from build123d import *

# Parameters (mm, degrees)
RESSALTO_EXTRUS_O2_DEPTH = 3
RESSALTO_EXTRUS_O3_DEPTH = 3
ESBO_O4_R                = 1.65
CORTE_EXTRUS_O2_DEPTH    = 55.465328173


with BuildPart() as part:
    # Esboço1 → Ressalto-extrusão2 (new body)
    with BuildSketch(Plane.XY):
        Polygon((-23.89, 48.854271798), (-23.89, 4.854271798), (-18.042684332, 4.854271798), (3.957315668, 4.854271798), (18.042684332, 4.854271798), (23.89, 4.854271798), (23.89, 48.854271798), align=None)
        Polygon((19.113248654, 42), (16.226497308, 47), (22, 47), (22, 42), align=None, mode=Mode.SUBTRACT)
        Polygon((-16.226497308, 8), (-22, 8), (-22, 13), (-19.113248654, 13), align=None, mode=Mode.SUBTRACT)
        Polygon((-8.113248654, 19.947441117), (-5.226497308, 14.947441117), (-8.113248654, 9.947441117), (-13.886751346, 9.947441117), (-16.773502692, 14.947441117), (-13.886751346, 19.947441117), align=None, mode=Mode.SUBTRACT)
        Polygon((-19.113248654, 16), (-22, 16), (-22, 26), (-19.113248654, 26), (-16.226497308, 21), align=None, mode=Mode.SUBTRACT)
        Polygon((-2.886751346, 13), (2.886751346, 13), (5.773502692, 8), (-5.773502692, 8), align=None, mode=Mode.SUBTRACT)
        Polygon((22, 8), (16.226497308, 8), (19.113248654, 13), (22, 13), align=None, mode=Mode.SUBTRACT)
        Polygon((13.886751346, 19.947441117), (16.773502692, 14.947441117), (13.886751346, 9.947441117), (8.113248654, 9.947441117), (5.226497308, 14.947441117), (8.113248654, 19.947441117), align=None, mode=Mode.SUBTRACT)
        Polygon((-2.886751346, 26), (2.886751346, 26), (5.773502692, 21), (2.886751346, 16), (-2.886751346, 16), (-5.773502692, 21), align=None, mode=Mode.SUBTRACT)
        Polygon((22, 16), (19.113248654, 16), (16.226497308, 21), (19.113248654, 26), (22, 26), align=None, mode=Mode.SUBTRACT)
        Polygon((-19.113248654, 29), (-22, 29), (-22, 39), (-19.113248654, 39), (-16.226497308, 34), align=None, mode=Mode.SUBTRACT)
        Polygon((-8.113248654, 33.044060566), (-5.226497308, 28.044060566), (-8.113248654, 23.044060566), (-13.886751346, 23.044060566), (-16.773502692, 28.044060566), (-13.886751346, 33.044060566), align=None, mode=Mode.SUBTRACT)
        Polygon((-19.113248654, 42), (-22, 42), (-22, 47), (-16.226497308, 47), align=None, mode=Mode.SUBTRACT)
        Polygon((-8.113248654, 46.140680015), (-5.226497308, 41.140680015), (-8.113248654, 36.140680015), (-13.886751346, 36.140680015), (-16.773502692, 41.140680015), (-13.886751346, 46.140680015), align=None, mode=Mode.SUBTRACT)
        Polygon((-2.886751346, 39), (2.886751346, 39), (5.773502692, 34), (2.886751346, 29), (-2.886751346, 29), (-5.773502692, 34), align=None, mode=Mode.SUBTRACT)
        Polygon((13.886751346, 32.995750841), (16.773502692, 27.995750841), (13.886751346, 22.995750841), (8.113248654, 22.995750841), (5.226497308, 27.995750841), (8.113248654, 32.995750841), align=None, mode=Mode.SUBTRACT)
        Polygon((19.113248654, 39), (22, 39), (22, 29), (19.113248654, 29), (16.226497308, 34), align=None, mode=Mode.SUBTRACT)
        Polygon((-5.801394324, 47.096619449), (5.801394324, 47.096619449), (2.858859713, 42), (-2.858859713, 42), align=None, mode=Mode.SUBTRACT)
        Polygon((13.886751346, 46.044060566), (16.773502692, 41.044060566), (13.886751346, 36.044060566), (8.113248654, 36.044060566), (5.226497308, 41.044060566), (8.113248654, 46.044060566), align=None, mode=Mode.SUBTRACT)
    extrude(amount=RESSALTO_EXTRUS_O2_DEPTH)

    # Esboço2 → Ressalto-extrusão3 (add)
    with BuildSketch(Plane.XY.offset(3)):
        Polygon((22.5, 48.854271798), (-22.5, 48.854271798), (-22.5, 42), (-16.5, 42), (-16.5, 47.096619449), (16.5, 47.096619449), (16.5, 42), (22.5, 42), align=None)
        Polygon((-22.5, 13), (-22.5, 4.854271798), (22.5, 4.854271798), (22.5, 13), (16.5, 13), (16.5, 8), (-16.5, 8), (-16.5, 13), align=None)
    extrude(amount=-RESSALTO_EXTRUS_O3_DEPTH)

    # Esboço4 → Corte-extrusão2 (cut, through all)
    with BuildSketch(Plane.XY.offset(3)):
        with Locations((-20.89, 45.854271798)):
            Circle(ESBO_O4_R)
        with Locations((-20.89, 7.854271798)):
            Circle(ESBO_O4_R)
        with Locations(Location((20.89, 7.854271798, 0), (0, 0, 180))):
            Circle(ESBO_O4_R)
        with Locations(Location((20.89, 45.854271798, 0), (0, 0, 180))):
            Circle(ESBO_O4_R)
    extrude(amount=-CORTE_EXTRUS_O2_DEPTH, mode=Mode.SUBTRACT)


solid = part.part
The model under review builds one solid part; all positions refer to its coordinate system, in mm. Coordinates: 2 decimals unless noted, no trailing zeros. Write each loop counter-clockwise with the first axis right and the second up, starting at its lowest first coordinate (ties: lowest second). Pieces come first, ordered by that corner, then holes. Notation, with made-up numbers: (53.25, -37.5) -> (102.25, -37.5) arc R25 cw to (102.25, -1.5) -> close; hole circle Ø1 at (72.25, -3). An arc over 180 degrees is marked (long way). Answer in a Markdown table with one row per item.
1. Wall thickness on probe 1 along Y at (x, z) = (-20.89, 2.4); probe 2 along Y at (x, z) = (-10, 0.95); probe 3 along Y at (x, z) = (11.5, 0.2): over which ranges is each line inside the solid? List them lowest first. Write a range as [from, to].
Answers below:
| item | result |
|---|---|
| probe 1 | y = [4.85, 6.2], [9.5, 16], [26, 29], [39, 44.2], [47.5, 48.85] |
| probe 2 | y = [4.85, 9.95], [19.95, 23.04], [33.04, 36.14], [46.14, 48.85] |
| probe 3 | y = [4.85, 9.95], [19.95, 23], [33, 36.04], [46.04, 48.85] |
2. Draft analysis for pull direction X (two halves, no side actions). For faces 1 (the flat face through (0, 4.854, 1)), 2 (the flat face through (-23.89, 27, 1)), 3 (the flat face through (-4.35, 23.465, 1.479)), state which applies: +X half, -X half, draft (parallel to the pull), parting line (faces both ways), or undercut.
Answers below:
| item | result |
|---|---|
| face 1 | draft |
| face 2 | -X half |
| face 3 | undercut |
3. Clearance check with a flat-ended pin moving along its axis: pin 1 Ø4 at (x, y) = (12, 39.5) entering from +Z. State where the tip first meets the part, or that it passes through.
Answers below:
| item | result |
|---|---|
| pin 1 | passes through |
4. We need section D-D, the plane y = 18. State the section outline as (x, z) points, and give its area (3 significant figures).
Answers below:
| item | result |
|---|---|
| outline | (-23.89, 0) -> (-22, 0) -> (-22, 3) -> (-23.89, 3) -> close; (-17.96, 0) -> (-15.01, 0) -> (-15.01, 3) -> (-17.96, 3) -> close; (-6.99, 0) -> (-4.04, 0) -> (-4.04, 3) -> (-6.99, 3) -> close; (4.04, 0) -> (6.99, 0) -> (6.99, 3) -> (4.04, 3) -> close; (15.01, 0) -> (17.96, 0) -> (17.96, 3) -> (15.01, 3) -> close; (22, 0) -> (23.89, 0) -> (23.89, 3) -> (22, 3) -> close |
| area | 46.7 mm^2 |
5. We need section C-C, the plane x = -7. State the section outline as (y, z) points, and give its area (3 significant figures).
Answers below:
| item | result |
|---|---|
| outline | (4.85, 0) -> (11.88, 0) -> (11.88, 3) -> (4.85, 3) -> close; (18.02, 0) -> (24.97, 0) -> (24.97, 3) -> (18.02, 3) -> close; (31.12, 0) -> (38.07, 0) -> (38.07, 3) -> (31.12, 3) -> close; (44.21, 0) -> (48.85, 0) -> (48.85, 3) -> (44.21, 3) -> close |
| area | 76.7 mm^2 |
6. We need section A-A, the plane x = 20.89. State the section outline as (y, z) points.
Answers below:
| item | result |
|---|---|
| outline | (4.85, 0) -> (6.2, 0) -> (6.2, 3) -> (4.85, 3) -> close; (9.5, 0) -> (16, 0) -> (16, 3) -> (9.5, 3) -> close; (26, 0) -> (29, 0) -> (29, 3) -> (26, 3) -> close; (39, 0) -> (44.2, 0) -> (44.2, 3) -> (39, 3) -> close; (47.5, 0) -> (48.85, 0) -> (48.85, 3) -> (47.5, 3) -> close |
7. We need section B-B, the plane y = 10.5. State the section outline as (x, z) points.
Answers below:
| item | result |
|---|---|
| outline | (-23.89, 0) -> (-14.21, 0) -> (-14.21, 3) -> (-23.89, 3) -> close; (-7.79, 0) -> (-4.33, 0) -> (-4.33, 3) -> (-7.79, 3) -> close; (4.33, 0) -> (7.79, 0) -> (7.79, 3) -> (4.33, 3) -> close; (14.21, 0) -> (23.89, 0) -> (23.89, 3) -> (14.21, 3) -> close |
